Source: CAD feature listing. Evaluate the final solid. Frame: model axes, mm. A direction names the side the tool comes from. Coordinates: 2 decimals unless noted, no trailing zeros. Order: outer loops, then holes, each group sorted by start corner. A loop starts at its lowest first (then second) coordinate and runs counter-clockwise, first axis right, second up. Notation, with made-up numbers: (16.25, 58.5) -> (71.25, 58.5) arc R31 cw to (71.25, 93.5) -> close; hole circle Ø9 at (16.5, 63). An arc over 180 degrees is marked (long way). Write item = value, one per line. Start each with the question number.
Item 1: Section query B-B (z = 4). Count the separate pieces of the cut face and the enclosed holes in it, then the cut area to 3 significant figures.
Item 2: Section query A-A (x = 40.5). Output: boundary loops of the cut face in (y, z).
Item 3: Section query C-C (y = 111.5). Output: boundary loops of the cut face in (x, z).
Item 4: Contact query for flat-ended pins moving along their axis: pin 1 (2 mm diameter, centred on x = 165.5, z = 25.5, fed in from +Y); pin 2 (6.5 mm diameter, centred on x = 108, y = 182, fed in from +Z); pin 3 (2 mm diameter, centred on x = 29, z = 27.5, fed in from +Y); pin 4 (1.5 mm diameter, centred on x = 69.5, y = 175.5, fed in from +Z). Output: stop coordinate, or through.
Item 5: Set-up query: faces 1 (the cylindrical face through (166.074, 102.436, 15.21)), 2 (the cylindrical face through (28.768, 174.507, 19.504)), 3 (the cylindrical face through (147.881, 122.848, 16.057)). Return all of +Z, -Z, +X, -X, +Y, -Y with unobstructed straight access to the full face (end or side cutting, diameter ignored); none if empty.
Item 6: Ray query, line 1 along Y through (x, z) = (152.5, 8); line 2 along Y through (x, z) = (130, 19); line 3 along X through (y, z) = (106, 26.75). Return the intervals inside material, ascending. Write a range as [from, to].
Item 7: Mould query, pull axis Y, two halves, no side actions, for faces 4 (the flat face through (113, 103, 30)), 5 (the flat face through (98, 200.933, 15)), 6 (the cylindrical face through (45.193, 185.369, 16.057)). Classes: released by +Y, released by -Y, zero draft, split by the parting line, or undercut.
```python
from build123d import *

# Parameters (mm, degrees)
F0_W          = 140
F0_H          = 100
F1_DEPTH      = 30
F2_T          = -2.5
F3_W          = 50
F3_H          = 12
F4_DEPTH      = 205.5
F5_R          = 5
F6_R          = 5
F7_R          = 3
F8_R          = 5
F9_DEPTH      = 27.5
F10_T         = 2
F10_T3_DEPTH  = 93
F10_T5_DEPTH  = 133
F10_T8_ANGLE  = 90.000000001
F10_T10_ANGLE = 90.000000001
F10_T12_ANGLE = 90.000000001
F10_T14_ANGLE = 90.000000001
F11_ANGLE     = 60
F12_ANGLE     = 30
F13_ANGLE     = 90


# Not quite as in the source:
# - a shell that OpenCascade refuses in one call is made with other operations: the cavity is built on its own and cut out


with BuildPart() as f1:
    # F0 (on Top) → F1 (new body)
    with BuildSketch(Plane.XY):
        with Locations((50, 0)):
            Rectangle(F0_W, F0_H)
    extrude(amount=F1_DEPTH)

    # F2
    f2_openings = [f1.faces().sort_by_distance(p)[0] for p in [
        (50, 0, 30),
    ]]
    offset(amount=F2_T, openings=f2_openings)

    # F3 (on face) → F4 (cut)
    with BuildSketch(Plane.YZ.offset(120)):
        with Locations((0, 24)):
            Rectangle(F3_W, F3_H)
    extrude(amount=-F4_DEPTH, mode=Mode.SUBTRACT)

    # F5
    f5_edges = [f1.edges().sort_by_distance(p)[0] for p in [
        (-18.75, 25, 18),
        (-18.75, -25, 18),
        (118.75, -25, 18),
        (118.75, 25, 18),
    ]]
    fillet(f5_edges, radius=F5_R)

    # F6
    f6_edges = [f1.edges().sort_by_distance(p)[0] for p in [
        (120, 50, 15),
        (-20, 50, 15),
        (-20, -50, 15),
        (120, -50, 15),
    ]]
    fillet(f6_edges, radius=F6_R)

    # F7
    f7_edges = [f1.edges().sort_by_distance(p)[0] for p in [
        (-17.5, -47.5, 16.25),
        (-17.5, 47.5, 16.25),
        (117.5, 47.5, 16.25),
        (117.5, -47.5, 16.25),
    ]]
    fillet(f7_edges, radius=F7_R)

    # F8 (on face) → F9 (join, through all)
    with BuildSketch(Plane.XY.offset(2.5)):
        with Locations((-5, -30)):
            Circle(F8_R)
        with Locations((40, -30)):
            Circle(F8_R)
        with Locations((100, -30)):
            Circle(F8_R)
        with Locations((100, 30)):
            Circle(F8_R)
        with Locations((40, 30)):
            Circle(F8_R)
        with Locations((-5, 30)):
            Circle(F8_R)
    extrude(amount=F9_DEPTH)

    # F10: shell of thickness 2, made by hand


with BuildPart() as f10_core1:
    # F10_t2: copy of F1
    add(f1.part)

    # the walls: a layer under each face that stays
    f10_faces = [f10_core1.faces().sort_by_distance(p)[0] for p in [
        (-10, -48.2142857143, 30),
        (117.5, 0, 16.25),
        (116.6213203436, -46.6213203436, 16.25),
        (118.75, -25, 26.5),
        (50, -47.5, 16.25),
        (120, 0, 15),
        (-16.6213203436, -46.6213203436, 16.25),
        (118.5355339059, -48.5355339059, 15),
        (-17.5, 0, 16.25),
        (50, -50, 15),
        (-18.75, -25, 26.5),
        (-18.5355339059, -48.5355339059, 15),
        (-20, 0, 15),
        (-10, 48.2142857143, 30),
        (116.6213203436, 46.6213203436, 16.25),
        (118.75, 25, 26.5),
        (50, 0, 2.5),
        (118.75, 23.5355339059, 19.4644660941),
        (118.75, 0, 18),
        (118.75, -23.5355339059, 19.4644660941),
        (118.5355339059, 48.5355339059, 15),
        (50, 0, 0),
        (-18.75, -23.5355339059, 19.4644660941),
        (-16.6213203436, 46.6213203436, 16.25),
        (-18.75, 0, 18),
        (-18.75, 23.5355339059, 19.4644660941),
        (-18.75, 25, 26.5),
        (-18.5355339059, 48.5355339059, 15),
        (50, 47.5, 16.25),
        (50, 50, 15),
        (-10, -30, 16.25),
        (35, -30, 16.25),
        (95, -30, 16.25),
        (-10, 30, 16.25),
        (35, 30, 16.25),
        (95, 30, 16.25),
    ]]
    thicken(f10_faces, amount=-F10_T, mode=Mode.SUBTRACT)

    # F10_s4 → F10_t3 (cut)
    with BuildSketch(Plane.XZ.offset(-46.5)):
        Polygon((117.48, 2.52), (119.5, 2.5), (119.5, 0.5), (117.5, 0.5), align=None)
        Polygon((-17.48, 2.52), (-19.5, 2.5), (-19.5, 0.5), (-17.5, 0.5), align=None)
    extrude(amount=F10_T3_DEPTH, mode=Mode.SUBTRACT)

    # F10_s6 → F10_t5 (cut)
    with BuildSketch(Plane.YZ.offset(-16.5)):
        Polygon((-47.48, 2.52), (-49.5, 2.5), (-49.5, 0.5), (-47.5, 0.5), align=None)
        Polygon((47.48, 2.52), (47.5, 0.5), (49.5, 0.5), (49.5, 2.5), align=None)
    extrude(amount=F10_T5_DEPTH, mode=Mode.SUBTRACT)

    # F10_s7 → F10_t8 (revolve, cut)
    with BuildSketch(Plane.XZ.offset(44.5)):
        Polygon((117.48, 2.52), (119.5, 2.5), (119.5, 0.5), (117.5, 0.5), align=None)
    revolve(axis=Axis((114.5, -44.5, 2.5), (0, 0, -1)), revolution_arc=F10_T8_ANGLE, mode=Mode.SUBTRACT)

    # F10_s9 → F10_t10 (revolve, cut)
    with BuildSketch(Plane.YZ.offset(-14.5)):
        Polygon((-47.48, 2.52), (-49.5, 2.5), (-49.5, 0.5), (-47.5, 0.5), align=None)
    revolve(axis=Axis((-14.5, -44.5, 2.5), (0, 0, -1)), revolution_arc=F10_T10_ANGLE, mode=Mode.SUBTRACT)

    # F10_s11 → F10_t12 (revolve, cut)
    with BuildSketch(Plane.XZ.offset(-44.5)):
        Polygon((117.48, 2.52), (119.5, 2.5), (119.5, 0.5), (117.5, 0.5), align=None)
    revolve(axis=Axis((114.5, 44.5, 2.5), (0, 0, 1)), revolution_arc=F10_T12_ANGLE, mode=Mode.SUBTRACT)

    # F10_s13 → F10_t14 (revolve, cut)
    with BuildSketch(Plane.XZ.offset(-44.5)):
        Polygon((-17.48, 2.52), (-17.5, 0.5), (-19.5, 0.5), (-19.5, 2.5), align=None)
    revolve(axis=Axis((-14.5, 44.5, 2.5), (0, 0, -1)), revolution_arc=F10_T14_ANGLE, mode=Mode.SUBTRACT)

    # F10_s15 → F10_t16 (revolve, cut)
    with BuildSketch(Plane.XZ.offset(30)):
        Polygon((0.02, 2.52), (0, 0.5), (-2, 0.5), (-2, 2.5), align=None)
    revolve(axis=Axis((-5, -30, 2.5), (0, 0, 1)), mode=Mode.SUBTRACT)

    # F10_s17 → F10_t18 (revolve, cut)
    with BuildSketch(Plane.XZ.offset(30)):
        Polygon((45.02, 2.52), (45, 0.5), (43, 0.5), (43, 2.5), align=None)
    revolve(axis=Axis((40, -30, 2.5), (0, 0, 1)), mode=Mode.SUBTRACT)

    # F10_s19 → F10_t20 (revolve, cut)
    with BuildSketch(Plane.XZ.offset(30)):
        Polygon((105.02, 2.52), (105, 0.5), (103, 0.5), (103, 2.5), align=None)
    revolve(axis=Axis((100, -30, 2.5), (0, 0, 1)), mode=Mode.SUBTRACT)

    # F10_s21 → F10_t22 (revolve, cut)
    with BuildSketch(Plane.XZ.offset(-30)):
        Polygon((0.02, 2.52), (0, 0.5), (-2, 0.5), (-2, 2.5), align=None)
    revolve(axis=Axis((-5, 30, 2.5), (0, 0, 1)), mode=Mode.SUBTRACT)

    # F10_s23 → F10_t24 (revolve, cut)
    with BuildSketch(Plane.XZ.offset(-30)):
        Polygon((45.02, 2.52), (45, 0.5), (43, 0.5), (43, 2.5), align=None)
    revolve(axis=Axis((40, 30, 2.5), (0, 0, 1)), mode=Mode.SUBTRACT)

    # F10_s25 → F10_t26 (revolve, cut)
    with BuildSketch(Plane.XZ.offset(-30)):
        Polygon((105.02, 2.52), (105, 0.5), (103, 0.5), (103, 2.5), align=None)
    revolve(axis=Axis((100, 30, 2.5), (0, 0, 1)), mode=Mode.SUBTRACT)


with BuildPart() as f1_1:
    add(f1.part)

    # what is left inside the walls is the cavity
    f10_cavity = [f10_core1.part.solids().sort_by_distance(p)[0] for p in [
        (-7.98, -30, 11.333333),
        (37.02, -30, 11.333333),
        (97.02, -30, 11.333333),
        (-7.98, 30, 11.333333),
        (37.02, 30, 11.333333),
        (97.02, 30, 11.333333),
    ]]
    add(f10_cavity, mode=Mode.SUBTRACT)


with BuildPart() as f1_2:
    # F11: moved
    add(f1_1.part.rotate(Axis((-5, 30, 2), (0, 0, 1)), F11_ANGLE))


with BuildPart() as f1_3:
    # F12: moved
    add(f1_2.part.rotate(Axis((47.5, 120.9326673974, 0.5), (0, 0, 1)), F12_ANGLE))


with BuildPart() as f1_4:
    # F13: moved
    add(f1_3.part.rotate(Axis((47.5, 120.9326673974, 0.5), (0, 0, 1)), F13_ANGLE))


solid = f1_4.part
```
Computed:
q1.separate_pieces = 7
q1.enclosed_holes = 7
q1.area = 1,460 mm^2
q2.outline = (100.93, 0) -> (200.93, 0) -> (200.93, 30) -> (198.43, 30) -> (198.43, 2.5) -> (103.43, 2.5) -> (103.43, 30) -> (100.93, 30) -> close
q3.outline = (27.5, 0) -> (167.5, 0) -> (167.5, 30) -> (165, 30) -> (165, 2.5) -> (30, 2.5) -> (30, 30) -> (27.5, 30) -> close
q4.pin_1 = 200.52
q4.pin_2 = 30
q4.pin_3 = 200.26
q4.pin_4 = 2.5
q5.face_1 = +Z, -Z, +X, -Y
q5.face_2 = +Z, +X, -X
q5.face_3 = +Z
q6.line_1 = [100.93, 103.43], [115.93, 117.93], [123.93, 125.93], [175.93, 177.93], [183.93, 185.93], [198.43, 200.93]
q6.line_2 = [100.93, 103.43], [198.43, 200.93]
q6.line_3 = [27.5, 30.03], [164.97, 167.5]
q7.face_4 = zero draft
q7.face_5 = released by +Y
q7.face_6 = undercut
